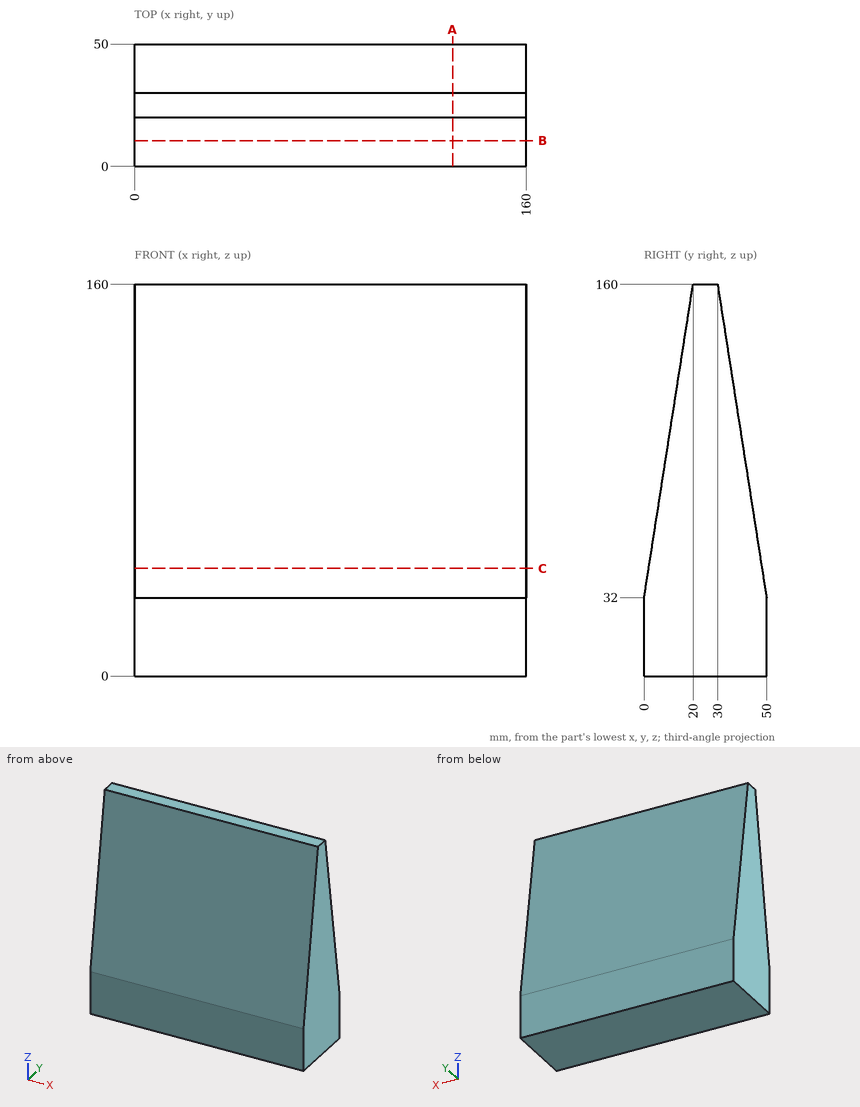
Input: dimensioned drawing with shaded views. Units: mm. Origin: part minimum x, y, z. Coordinates: 2 decimals unless noted, no trailing zeros. Order: outer loops, then holes, each group sorted by start corner. A loop starts at its lowest first (then second) coordinate and runs counter-clockwise, first axis right, second up. Notation, with made-up numbers: (19.5, 3.5) - (27.5, 3.5) arc R8 ccw to (27.5, 18.5) - close; hole circle Ø6 at (-9, 74). An arc over 180 degrees is marked (long way). Put each result on its own line as item: value.
1. Line query: line 1 along Y through (x, z) = (48.5, 94.5); line 2 along Y through (x, z) = (11, 68.5). Output: solid intervals per line, ascending.
Report:
line 1: y = 9.77 to 40.23
line 2: y = 5.7 to 44.3
2. Cut plane B-B on y = 10.5. Return the cut outline in (x, z), then the cut area to 3 significant figures.
Report:
outline: (0, 0) - (160, 0) - (160, 99.2) - (0, 99.2) - close
area: 15,900 mm2
3. Cut plane C-C on z = 44. Return the cut outline in (x, y) (3 decimals), then the cut area to 3 significant figures.
Report:
outline: (0, 1.875) - (160, 1.875) - (160, 48.125) - (0, 48.125) - close
area: 7,400 mm2
4. Cut plane A-A on x = 130. Return the cut outline in (y, z), then the cut area to 3 significant figures.
Report:
outline: (0, 0) - (50, 0) - (50, 32) - (30, 160) - (20, 160) - (0, 32) - close
area: 5,440 mm2
